Design review of the part built by this model. Coordinates are the model's own, in mm. Coordinates: 2 decimals unless noted, no trailing zeros. Loops run counter-clockwise (first coordinate to the right, second up) from the corner with the lowest first, then second, coordinate; pieces in that order, holes last. Notation, with made-up numbers: M -15,54 L 4,54 A18 ccw 4,79 Z; hole C 55,79 d3. An arc over 180 degrees is marked long. One line per item, written item: value.
```python
from build123d import *

# Parameters (mm, degrees)
BASE_FLANGE1_DEPTH = 0.8


# Sheet-metal steps are written as plain solids
with BuildPart() as part:
    # Sketch1 → Base-Flange1 (new body)
    with BuildSketch(Plane(origin=(0, 0, 0), x_dir=(1, 0, 0), z_dir=(0, 1, 0))):
        with BuildLine():
            Line((-455.05, -59), (333.35, -59))
            Line((333.35, -59), (333.35, -19))
            Line((333.35, -19), (374.15, -19))
            Line((374.15, -19), (374.15, -16))
            ThreePointArc((374.15, -16), (352.183008589, 37.033008589), (299.15, 59))
            Line((299.15, 59), (-420.85, 59))
            ThreePointArc((-420.85, 59), (-473.883008589, 37.033008589), (-495.85, -16))
            Line((-495.85, -16), (-495.85, -19))
            Line((-495.85, -19), (-455.05, -19))
            Line((-455.05, -19), (-455.05, -59))
        make_face()
    extrude(amount=-BASE_FLANGE1_DEPTH)


solid = part.part
```
(1) Insertion check: pin 1 (4 mm diameter, centred on x = -125, z = -45, fed in from +Y). The pin has a flat end and moves straight along its axis. Give the tip position at first contact, or say it passes through.
Reply:
pin 1: stops at y = 0
(2) We need section C-C on z = -19.5. State the section outline as (x, y) points, then the cut area to 3 significant figures.
Reply:
outline: M -486.92,-0.8 L 365.22,-0.8 L 365.22,0 L -486.92,0 Z
area: 682 mm2
(3) We need section A-A on y = -0.6. State the section outline as (x, z) points, then the cut area to 3 significant figures.
Reply:
outline: M -495.85,16 A75 ccw -420.85,-59 L 299.15,-59 A75 ccw 374.15,16 L 374.15,19 L 333.35,19 L 333.35,59 L -455.05,59 L -455.05,19 L -495.85,19 Z
area: 97,000 mm2
(4) We need section B-B on z = 48.5. State the section outline as (x, y) points, then the cut area to 3 significant figures.
Reply:
outline: M -455.05,-0.8 L 333.35,-0.8 L 333.35,0 L -455.05,0 Z
area: 631 mm2
(5) To check wall thickness, follow line 1 along X through (y, z) = (-0.7, 52); line 2 along X through (y, z) = (-0.4, 14); line 3 along Z through (x, y) = (312, -0.45). State the ranges of each line that lie inside material, in increasing order. Write a range as [from, to].
Reply:
line 1: x = [-455.05, 333.35]
line 2: x = [-495.82, 374.12]
line 3: z = [-57.89, 59]
